Can you work these out from the drawing? Everything is in mm from the part's minimum corner. A direction names the side the tool comes from. Give positions to 0.01 mm unless a question says otherwise; leave off trailing zeros. Write each loop counter-clockwise with the first axis right and the second up, starting at its lowest first coordinate (ties: lowest second). Pieces come first, ordered by that corner, then holes. Notation, with made-up numbers: M 31,34 L 37,34 A4 cw 37,41 Z; hole C 9,-20 d5. An arc over 180 degrees is marked long. One line per item, written item: value.
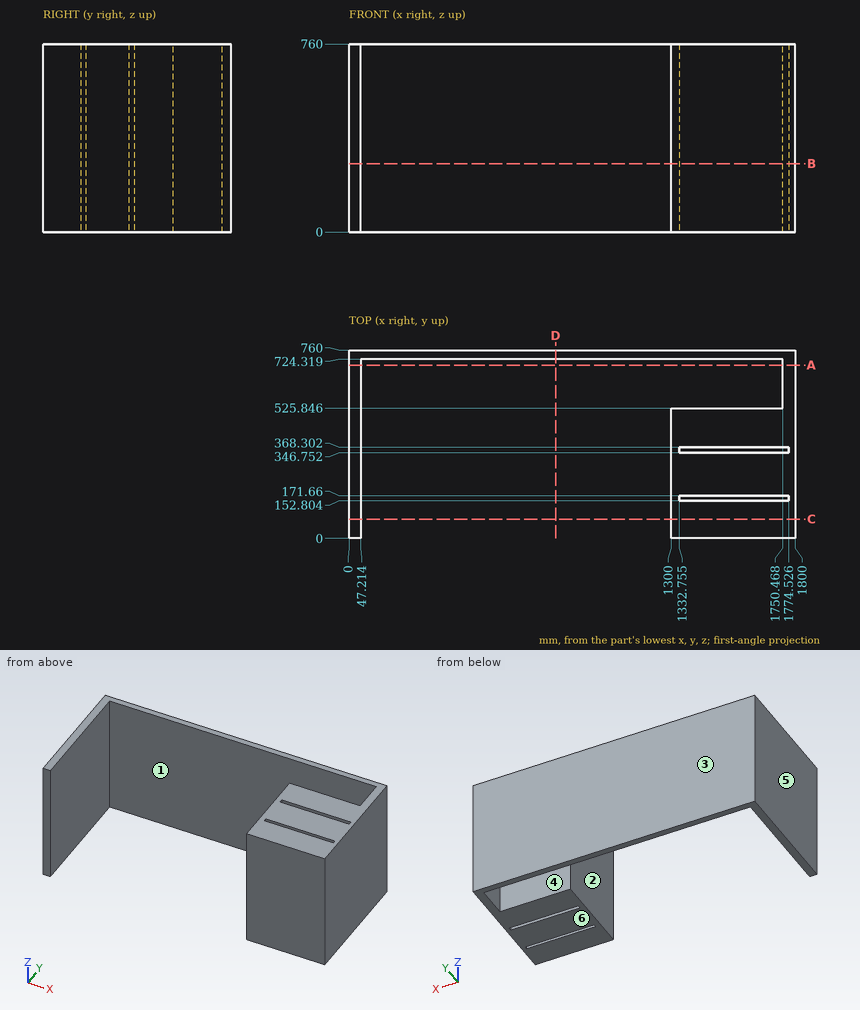
1) Please list where these lines run through material, in increasing order: L1, parallel to Y at x = 1387.5, z = 361 (1 decimal); L2, parallel to X at y = 349, z = 332 (1 decimal); L3, parallel to X at y = 682, z = 543.5. Write a range as from..to.
Outcome:
L1: y = 0..152.8, 171.7..346.8, 368.3..525.8, 724.3..760
L2: x = 0..47.2, 1300..1332.8, 1774.5..1800
L3: x = 0..47.21, 1750.47..1800
2) On a 3-axis mill with a long thin cutter (end or side, diameter ignored), from which of +Z, -Z, +X, -X, +Y, -Y can I reach the whole of each face in a straight line? I mean the marked faces 1, 2 and 3. Say none if no direction works.
Outcome:
face 1: +Z, -Z
face 2: +Z, -Z, -Y
face 3: +Z, -Z, +X, -X, +Y
3) If we section it at D-D, the plane x = 833: Write out the boundary of the cut face in (y, z).
Outcome:
outline: M 724.32,0 L 760,0 L 760,760 L 724.32,760 Z
4) If we section it at C-C, the plane y = 78: Write out the boundary of the cut face in (x, z), then the cut area to 3 significant figures.
Outcome:
outline: M 0,0 L 47.21,0 L 47.21,760 L 0,760 Z; M 1300,0 L 1800,0 L 1800,760 L 1300,760 Z
area: 416,000 mm^2
5) I'm going to push a flat-ended pin straight in: pin 1 (8 mm diameter, centred on x = 584, z = 308.5, fed in from -Y). Where does the tip first touch, or does it pass through?
Outcome:
pin 1: stops at y = 724.32
6) We'd pull the mould along X, two halves only. Please class the marked faces 4, 5 and 6: pulls with the +X half, pulls with the -X half, needs draft (parallel to the pull), parting line crosses it, or undercut.
Outcome:
face 4: undercut
face 5: pulls with the -X half
face 6: needs draft
7) If we section it at B-B, the plane z = 277: Write out the boundary of the cut face in (x, y) (1 decimal), then the cut area to 3 significant figures.
Outcome:
outline: M 0,0 L 47.2,0 L 47.2,724.3 L 1750.5,724.3 L 1750.5,525.8 L 1300,525.8 L 1300,0 L 1800,0 L 1800,760 L 0,760 Z; hole M 1332.8,152.8 L 1774.5,152.8 L 1774.5,171.7 L 1332.8,171.7 Z; hole M 1332.8,346.8 L 1774.5,346.8 L 1774.5,368.3 L 1332.8,368.3 Z
area: 353,000 mm^2
8) If we section it at A-A, the plane y = 699.5: Write out the boundary of the cut face in (x, z).
Outcome:
outline: M 0,0 L 47.21,0 L 47.21,760 L 0,760 Z; M 1750.47,0 L 1800,0 L 1800,760 L 1750.47,760 Z
